from build123d import *

# Parameters (mm, degrees)
SKETCH1_W           = 60
SKETCH1_H           = 24
BOSS_EXTRUDE1_DEPTH = 3.3
SKETCH2_W           = 3.3
SKETCH2_H           = 24
BOSS_EXTRUDE2_DEPTH = 61.3
SKETCH3_W           = 16
SKETCH3_H           = 31.8
CUT_EXTRUDE1_DEPTH  = 3.3
CUT_EXTRUDE2_DEPTH  = 3.3
SKETCH5_R           = 4.5
SKETCH5_R_2         = 1.5
CUT_EXTRUDE3_DEPTH  = 3.3
SKETCH7_R           = 1.5
SKETCH7_W           = 29.4
SKETCH7_H           = 14
CUT_EXTRUDE4_DEPTH  = 3.3
FILLET1_R           = 3


with BuildPart() as part:
    # Sketch1 → Boss-Extrude1 (new body)
    with BuildSketch(Plane(origin=(0, 0, 0), x_dir=(1, 0, 0), z_dir=(0, 1, 0))):
        Rectangle(SKETCH1_W, SKETCH1_H)
    extrude(amount=BOSS_EXTRUDE1_DEPTH)

    # Sketch2 → Boss-Extrude2 (add)
    with BuildSketch(Plane(origin=(0, 0, 0), x_dir=(1, 0, 0), z_dir=(0, 1, 0))):
        with Locations((28.35, 0)):
            Rectangle(SKETCH2_W, SKETCH2_H)
    boss_extrude2 = extrude(amount=BOSS_EXTRUDE2_DEPTH)

    # Sketch3 → Cut-Extrude1 (cut)
    with BuildSketch(Plane(origin=(30, 0, 0), x_dir=(0, 0, -1), z_dir=(1, 0, 0))):
        with Locations((0, 25.9)):
            Rectangle(SKETCH3_W, SKETCH3_H)
    cut_extrude1 = extrude(amount=-CUT_EXTRUDE1_DEPTH, mode=Mode.SUBTRACT)

    # Sketch4 → Cut-Extrude2 (cut)
    with BuildSketch(Plane(origin=(30, 0, 0), x_dir=(0, 0, -1), z_dir=(1, 0, 0))):
        with BuildLine():
            ThreePointArc((2.4e-08, 61.3), (8.485281383, 57.785281366), (12, 49.3))
            Line((12, 49.3), (12, 61.3))
            Line((12, 61.3), (2.4e-08, 61.3))
        make_face()
        with BuildLine():
            ThreePointArc((-12, 49.3), (-8.485281366, 57.785281383), (2.4e-08, 61.3))
            Line((2.4e-08, 61.3), (-12, 61.3))
            Line((-12, 61.3), (-12, 49.3))
        make_face()
    cut_extrude2 = extrude(amount=-CUT_EXTRUDE2_DEPTH, mode=Mode.SUBTRACT)

    # Sketch5 → Cut-Extrude3 (cut)
    with BuildSketch(Plane(origin=(30, 0, 0), x_dir=(0, 0, -1), z_dir=(1, 0, 0))):
        with Locations((0, 49.3)):
            Circle(SKETCH5_R)
        with Locations((8.4, 49.3)):
            Circle(SKETCH5_R_2)
        with Locations((0, 57.7)):
            Circle(SKETCH5_R_2)
        with Locations((-8.4, 49.3)):
            Circle(SKETCH5_R_2)
    cut_extrude3 = extrude(amount=-CUT_EXTRUDE3_DEPTH, mode=Mode.SUBTRACT)

    # Sketch7 → Cut-Extrude4 (cut)
    with BuildSketch(Plane(origin=(0, 0, 0), x_dir=(1, 0, 0), z_dir=(0, 1, 0))):
        with Locations((-21.3, 0)):
            Circle(SKETCH7_R)
        with Locations((14.7, 0)):
            Circle(SKETCH7_R)
        with Locations((-3.3, 0)):
            Rectangle(SKETCH7_W, SKETCH7_H)
    extrude(amount=CUT_EXTRUDE4_DEPTH, mode=Mode.SUBTRACT)

    # Mirror2: Boss-Extrude2, Cut-Extrude1, Cut-Extrude2, Cut-Extrude3 across plane
    add(boss_extrude2.mirror(Plane(origin=(0, 0, 0), x_dir=(0, 0, 1), z_dir=(1, 0, 0))))
    add(cut_extrude1.mirror(Plane(origin=(0, 0, 0), x_dir=(0, 0, 1), z_dir=(1, 0, 0))), mode=Mode.SUBTRACT)
    add(cut_extrude2.mirror(Plane(origin=(0, 0, 0), x_dir=(0, 0, 1), z_dir=(1, 0, 0))), mode=Mode.SUBTRACT)
    add(cut_extrude3.mirror(Plane(origin=(0, 0, 0), x_dir=(0, 0, 1), z_dir=(1, 0, 0))), mode=Mode.SUBTRACT)

    # Fillet1
    fillet1_edges = [part.edges().sort_by_distance(p)[0] for p in [
        (-26.7, 3.3, 0),
        (-28.35, 10, 8),
        (-28.35, 41.8, 8),
        (-28.35, 41.8, -8),
        (-28.35, 10, -8),
        (26.7, 3.3, 0),
        (28.35, 41.8, -8),
        (28.35, 10, -8),
        (28.35, 10, 8),
        (28.35, 41.8, 8),
        (-30, 0, 0),
        (30, 0, 0),
    ]]
    fillet(fillet1_edges, radius=FILLET1_R)


solid = part.part
The model under review builds one solid part; all positions refer to its coordinate system, in mm. A direction names the side the tool comes from. Coordinates: 2 decimals unless noted, no trailing zeros. Write each loop counter-clockwise with the first axis right and the second up, starting at its lowest first coordinate (ties: lowest second). Pieces come first, ordered by that corner, then holes. Notation, with made-up numbers: (45.5, -36.75) - (97.5, -36.75) arc R30 ccw to (97.5, -10.75) - close; hole circle Ø7 at (-18, 13.25). An arc over 180 degrees is marked (long way). Answer as a JSON object with one key per item and string values. Group by question number.
1. Add section D-D (x = 14.7). Give the boundary of the cut face in (y, z), plus the area to 3 significant figures.
2. Mouldability with a two-part tool opening along X and no side actions: class faces 1 (the face through (-30, 31.7, 8.2)), 2 (the face through (-28.37, 47.97, 7.71)), 3 (the face through (-18, 2, 0)), 4 (the face through (-26.7, 33.4, 8.2)) as pulls with the +X half, pulls with the -X half, needs draft (parallel to the pull), parting line crosses it, or undercut.
3. Add section A-A (x = -2). Give the boundary of the cut face in (y, z).
4. Add section B-B (y = 15). Give the boundary of the cut face in (x, z), plus the area to 3 significant figures.
5. To check wall thickness, follow probe 1 along X at (y, z) = (44, -5.5); probe 2 along Z at (x, y) = (27, 49); probe 3 along Y at (x, z) = (22, 10). State the ranges of each line that lie inside material, in increasing order.
6. Clearance check with flat-ended pins moving along their axes: pin 1 Ø1 at (y, z) = (2.5, 0.5) entering from -X; pin 2 Ø7 at (x, z) = (11.5, -2.5) entering from +Y; pin 3 Ø2.5 at (x, z) = (28.5, 0.5) entering from -Y; pin 4 Ø2.5 at (x, z) = (28.5, 1.5) entering from +Y. State where each tip first meets the part, or that it passes through.
7. Add section C-C (z = -3.25). Give the number of separate pieces and of enclosed holes in the cut face, plus the area to 3 significant figures.
8. Machinability: for faces 5 (the face through (26.7, 33.4, 8.2)), 6 (the face through (-29.1, 0.86, -0.17)), 7 (the face through (-28.33, 40.94, -7.1)), which of the approach directions +Z, -Z, +X, -X, +Y, -Y give a long, thin tool a straight path to every point of the face, cutting with its end or side? Answer none if there is none.
Findings:
{
 "1": {"outline": "(0, -12) - (3.3, -12) - (3.3, -1.5) - (0, -1.5) - close; (0, 1.5) - (3.3, 1.5) - (3.3, 12) - (0, 12) - close", "area": "69.3 mm²"},
 "2": {"face 1": "pulls with the -X half", "face 2": "needs draft", "face 3": "undercut", "face 4": "undercut"},
 "3": {"outline": "(0, -12) - (3.3, -12) - (3.3, -7) - (0, -7) - close; (0, 7) - (3.3, 7) - (3.3, 12) - (0, 12) - close"},
 "4": {"outline": "(-30, -12) - (-26.7, -12) - (-26.7, -8) - (-30, -8) - close; (-30, 8) - (-26.7, 8) - (-26.7, 12) - (-30, 12) - close; (26.7, -12) - (30, -12) - (30, -8) - (26.7, -8) - close; (26.7, 8) - (30, 8) - (30, 12) - (26.7, 12) - close", "area": "52.8 mm²"},
 "5": {"probe 1": "-30 to -26.7, 26.7 to 30", "probe 2": "-12 to -9.87, -6.93 to -4.49, 4.49 to 6.93, 9.87 to 12", "probe 3": "0 to 3.3"},
 "6": {"pin 1": "x = -30", "pin 2": "y = 3.3", "pin 3": "y = 0.01", "pin 4": "y = 61.3"},
 "7": {"separate pieces": "6", "enclosed holes": "0", "area": "230 mm²"},
 "8": {"face 5": "+Z, -Z, +Y", "face 6": "+Z, -Z, -X, -Y", "face 7": "+X, -X"}
}
